```python
from build123d import *

# Parameters (mm, degrees)
SKETCH1_W           = 15
SKETCH1_H           = 185.68
SKETCH1_R           = 2.895
SKETCH1_W_2         = 343.08
SKETCH1_H_2         = 25
SKETCH1_H_3         = 15
BOSS_EXTRUDE1_DEPTH = 8
SKETCH2_W           = 15
SKETCH2_H           = 10
BOSS_EXTRUDE2_DEPTH = 100
SKETCH3_R           = 2
BOSS_EXTRUDE3_DEPTH = 4
CUT_EXTRUDE1_REACH  = 367.547
SKETCH5_R           = 1.35
BOSS_EXTRUDE4_DEPTH = 5


with BuildPart() as part:
    # Sketch1 → Boss-Extrude1 (new body)
    # profile 1 of 11: a face of its own
    with BuildSketch(Plane(origin=(0, 0, 0), x_dir=(1, 0, 0), z_dir=(0, 1, 0))):
        with Locations((-7.5, 92.84)):
            Rectangle(SKETCH1_W, SKETCH1_H)
        with Locations(Location((-7.5, 6.7, 0), (0, 0, 270))):
            Circle(SKETCH1_R, mode=Mode.SUBTRACT)
        with Locations(Location((-7.5, 178.98, 0), (0, 0, 270))):
            Circle(SKETCH1_R, mode=Mode.SUBTRACT)
    # profile 2 of 11: a face of its own
    with BuildSketch(Plane(origin=(0, 0, 0), x_dir=(1, 0, 0), z_dir=(0, 1, 0))):
        with Locations((-32.89, 92.84)):
            Rectangle(SKETCH1_W, SKETCH1_H)
        with Locations(Location((-32.89, 6.7, 0), (0, 0, 270))):
            Circle(SKETCH1_R, mode=Mode.SUBTRACT)
        with Locations(Location((-32.89, 178.98, 0), (0, 0, 270))):
            Circle(SKETCH1_R, mode=Mode.SUBTRACT)
    # profile 3 of 11: a face of its own
    with BuildSketch(Plane(origin=(0, 0, 0), x_dir=(1, 0, 0), z_dir=(0, 1, 0))):
        with Locations((-72.88, 92.84)):
            Rectangle(SKETCH1_W, SKETCH1_H)
        with Locations(Location((-72.88, 6.7, 0), (0, 0, 270))):
            Circle(SKETCH1_R, mode=Mode.SUBTRACT)
        with Locations(Location((-72.88, 178.98, 0), (0, 0, 270))):
            Circle(SKETCH1_R, mode=Mode.SUBTRACT)
    # profile 4 of 11: a face of its own
    with BuildSketch(Plane(origin=(0, 0, 0), x_dir=(1, 0, 0), z_dir=(0, 1, 0))):
        with Locations((-112.87, 92.84)):
            Rectangle(SKETCH1_W, SKETCH1_H)
        with Locations(Location((-112.87, 6.7, 0), (0, 0, 270))):
            Circle(SKETCH1_R, mode=Mode.SUBTRACT)
        with Locations(Location((-112.87, 178.98, 0), (0, 0, 270))):
            Circle(SKETCH1_R, mode=Mode.SUBTRACT)
    # profile 5 of 11: a face of its own
    with BuildSketch(Plane(origin=(0, 0, 0), x_dir=(1, 0, 0), z_dir=(0, 1, 0))):
        with Locations((-157.74, 52.84)):
            Rectangle(SKETCH1_W_2, SKETCH1_H_2)
        with Locations(Location((-157.74, 52.84, 0), (0, 0, 270))):
            Circle(SKETCH1_R, mode=Mode.SUBTRACT)
    # profile 6 of 11: a face of its own
    with BuildSketch(Plane(origin=(0, 0, 0), x_dir=(1, 0, 0), z_dir=(0, 1, 0))):
        with Locations((-157.74, 92.84)):
            Rectangle(SKETCH1_W_2, SKETCH1_H_3)
        with Locations(Location((7.1, 92.84, 0), (0, 0, 270))):
            Circle(SKETCH1_R, mode=Mode.SUBTRACT)
        with Locations(Location((-157.74, 92.84, 0), (0, 0, 270))):
            Circle(SKETCH1_R, mode=Mode.SUBTRACT)
        with Locations(Location((-322.58, 92.84, 0), (0, 0, 270))):
            Circle(SKETCH1_R, mode=Mode.SUBTRACT)
    # profile 7 of 11: a face of its own
    with BuildSketch(Plane(origin=(0, 0, 0), x_dir=(1, 0, 0), z_dir=(0, 1, 0))):
        with Locations((-157.74, 132.84)):
            Rectangle(SKETCH1_W_2, SKETCH1_H_2)
        with Locations(Location((-157.74, 132.84, 0), (0, 0, 270))):
            Circle(SKETCH1_R, mode=Mode.SUBTRACT)
    # profile 8 of 11: a face of its own
    with BuildSketch(Plane(origin=(0, 0, 0), x_dir=(1, 0, 0), z_dir=(0, 1, 0))):
        with Locations((-202.61, 92.84)):
            Rectangle(SKETCH1_W, SKETCH1_H)
        with Locations(Location((-202.61, 178.98, 0), (0, 0, 270))):
            Circle(SKETCH1_R, mode=Mode.SUBTRACT)
        with Locations(Location((-202.61, 6.7, 0), (0, 0, 270))):
            Circle(SKETCH1_R, mode=Mode.SUBTRACT)
    # profile 9 of 11: a face of its own
    with BuildSketch(Plane(origin=(0, 0, 0), x_dir=(1, 0, 0), z_dir=(0, 1, 0))):
        with Locations((-242.6, 92.84)):
            Rectangle(SKETCH1_W, SKETCH1_H)
        with Locations(Location((-242.6, 178.98, 0), (0, 0, 270))):
            Circle(SKETCH1_R, mode=Mode.SUBTRACT)
        with Locations(Location((-242.6, 6.7, 0), (0, 0, 270))):
            Circle(SKETCH1_R, mode=Mode.SUBTRACT)
    # profile 10 of 11: a face of its own
    with BuildSketch(Plane(origin=(0, 0, 0), x_dir=(1, 0, 0), z_dir=(0, 1, 0))):
        with Locations((-282.59, 92.84)):
            Rectangle(SKETCH1_W, SKETCH1_H)
        with Locations(Location((-282.59, 178.98, 0), (0, 0, 270))):
            Circle(SKETCH1_R, mode=Mode.SUBTRACT)
        with Locations(Location((-282.59, 6.7, 0), (0, 0, 270))):
            Circle(SKETCH1_R, mode=Mode.SUBTRACT)
    # profile 11 of 11: a face of its own
    with BuildSketch(Plane(origin=(0, 0, 0), x_dir=(1, 0, 0), z_dir=(0, 1, 0))):
        with Locations((-307.98, 92.84)):
            Rectangle(SKETCH1_W, SKETCH1_H)
        with Locations(Location((-307.98, 178.98, 0), (0, 0, 270))):
            Circle(SKETCH1_R, mode=Mode.SUBTRACT)
        with Locations(Location((-307.98, 6.7, 0), (0, 0, 270))):
            Circle(SKETCH1_R, mode=Mode.SUBTRACT)
    extrude(amount=BOSS_EXTRUDE1_DEPTH)

    # Sketch2 → Boss-Extrude2 (add)
    with BuildSketch(Plane(origin=(0, 8, 0), x_dir=(1, 0, 0), z_dir=(0, 1, 0))):
        with Locations((6.3, 60.34)):
            Rectangle(SKETCH2_W, SKETCH2_H)
        with Locations((-73.7, 60.34)):
            Rectangle(SKETCH2_W, SKETCH2_H)
    extrude(amount=BOSS_EXTRUDE2_DEPTH)

    # Sketch3 → Boss-Extrude3 (add)
    with BuildSketch(Plane(origin=(0, 0, -65.34), x_dir=(-1, 0, 0), z_dir=(0, 0, -1))):
        with Locations(Location((-7.8, 103.1, 0), (0, 0, 180))):
            Circle(SKETCH3_R)
        with Locations(Location((-7.8, 26.15, 0), (0, 0, 180))):
            Circle(SKETCH3_R)
        with Locations(Location((72.2, 26.15, 0), (0, 0, 180))):
            Circle(SKETCH3_R)
        with Locations(Location((72.2, 103.1, 0), (0, 0, 180))):
            Circle(SKETCH3_R)
    extrude(amount=BOSS_EXTRUDE3_DEPTH)

    # Sketch5 → Cut-Extrude1 (cut, up to next)
    with BuildSketch(Plane(origin=(0, 0, -69.34), x_dir=(-1, 0, 0), z_dir=(0, 0, -1)), mode=Mode.PRIVATE) as cut_extrude1_sk1:
        with Locations((-7.8, 103.1)):
            Circle(SKETCH5_R)
    cut_extrude1_tool1 = extrude(cut_extrude1_sk1.sketch, amount=-CUT_EXTRUDE1_REACH, mode=Mode.PRIVATE) & part.part
    # Sketch5 → Cut-Extrude1 (cut, up to next)
    with BuildSketch(Plane(origin=(0, 0, -69.34), x_dir=(-1, 0, 0), z_dir=(0, 0, -1)), mode=Mode.PRIVATE) as cut_extrude1_sk2:
        with Locations((-7.8, 26.15)):
            Circle(SKETCH5_R)
    cut_extrude1_tool2 = extrude(cut_extrude1_sk2.sketch, amount=-CUT_EXTRUDE1_REACH, mode=Mode.PRIVATE) & part.part
    # Sketch5 → Cut-Extrude1 (cut, up to next)
    with BuildSketch(Plane(origin=(0, 0, -69.34), x_dir=(-1, 0, 0), z_dir=(0, 0, -1)), mode=Mode.PRIVATE) as cut_extrude1_sk3:
        with Locations((72.2, 26.15)):
            Circle(SKETCH5_R)
    cut_extrude1_tool3 = extrude(cut_extrude1_sk3.sketch, amount=-CUT_EXTRUDE1_REACH, mode=Mode.PRIVATE) & part.part
    # Sketch5 → Cut-Extrude1 (cut, up to next)
    with BuildSketch(Plane(origin=(0, 0, -69.34), x_dir=(-1, 0, 0), z_dir=(0, 0, -1)), mode=Mode.PRIVATE) as cut_extrude1_sk4:
        with Locations((72.2, 103.1)):
            Circle(SKETCH5_R)
    cut_extrude1_tool4 = extrude(cut_extrude1_sk4.sketch, amount=-CUT_EXTRUDE1_REACH, mode=Mode.PRIVATE) & part.part
    add(cut_extrude1_tool1.solids().sort_by_distance((7.8, 103.1, -69.34))[0], mode=Mode.SUBTRACT)
    add(cut_extrude1_tool2.solids().sort_by_distance((7.8, 26.15, -69.34))[0], mode=Mode.SUBTRACT)
    add(cut_extrude1_tool3.solids().sort_by_distance((-72.2, 26.15, -69.34))[0], mode=Mode.SUBTRACT)
    add(cut_extrude1_tool4.solids().sort_by_distance((-72.2, 103.1, -69.34))[0], mode=Mode.SUBTRACT)

    # Sketch7 → Boss-Extrude4 (add)
    with BuildSketch(Plane.ZY.offset(1.2)):
        Polygon((-40.34, 8), (-55.34, 108), (-55.34, 8), align=None)
    extrude(amount=-BOSS_EXTRUDE4_DEPTH)


solid = part.part
```
Geometry check sheet. Reference: the model listing, model coordinates, mm. A direction names the side the tool comes from. Round coordinates to 2 decimals unless told otherwise and drop trailing zeros. Loops run counter-clockwise (first coordinate to the right, second up) from the corner with the lowest first, then second, coordinate; pieces in that order, holes last. Notation, with made-up numbers: (56, 57.5) -> (70, 57.5) arc R27 cw to (70, 73.5) -> close; hole circle Ø1 at (19.25, 23.5). An arc over 180 degrees is marked (long way). Use a Markdown table: item, result.
(1) Sectioned sample at B-B (z = -158.5). Give the number of separate pieces and of enclosed holes in the cut face, then the cut area to 3 significant figures.
Calculated:
| item | result |
|---|---|
| separate pieces | 8 |
| enclosed holes | 0 |
| area | 960 mm² |
(2) Go/stop test with flat-tipped pins: P1, Ø4, axis at x = -151, y = 5.5, coming from the -Z side; P2, Ø4.5, axis at x = 8, y = 102.5, coming from the -Z side; P3, Ø4, axis at x = -144.5, y = 3.5, coming from the +Z side. Record where each tip stops, or that it passes through.
Calculated:
| item | result |
|---|---|
| P1 | z = -145.34 |
| P2 | z = -69.34 |
| P3 | z = -40.34 |
(3) Scan lines: probe 1 along Y at (x, z) = (-72, -62); probe 2 along Z at (x, y) = (-157.74, 6.25) (3 decimals); probe 3 along X at (y, z) = (4.75, -92.84) (3 decimals). Record each from-to range of solid material in increasing order.
Calculated:
| item | result |
|---|---|
| probe 1 | 0 to 24.81, 27.49 to 101.76, 104.44 to 108 |
| probe 2 | -145.34 to -135.735, -129.945 to -120.34, -100.34 to -95.735, -89.945 to -85.34, -65.34 to -55.735, -49.945 to -40.34 |
| probe 3 | -329.28 to -325.475, -319.685 to -160.635, -154.845 to 4.205, 9.995 to 13.8 |
(4) Sectioned sample at C-C (x = -93). Enter the section's corners in (y, z).
Calculated:
| item | result |
|---|---|
| outline | (0, -145.34) -> (8, -145.34) -> (8, -120.34) -> (0, -120.34) -> close; (0, -100.34) -> (8, -100.34) -> (8, -85.34) -> (0, -85.34) -> close; (0, -65.34) -> (8, -65.34) -> (8, -40.34) -> (0, -40.34) -> close |
(5) Set-up check for faces 1 (the flat face through (-105.37, 4, -110)), 2 (the flat face through (-93, 4, -40.34)), 3 (the flat face through (-66.2, 57, -60)): record each of +Z, -Z, +X, -X, +Y, -Y from which the full face is reachable in a straight line by a thin tool's end or side.
Calculated:
| item | result |
|---|---|
| face 1 | +Y, -Y |
| face 2 | +Z, +Y, -Y |
| face 3 | +Z, -Z, +Y |
(6) Mould release check, pull along Z, two halves, no side actions. Record for faces 4 (the flat face through (-80.38, 4, -75)), 5 (the flat face through (-113, 4, 0)), 6 (the flat face through (-73, 4, -185.68)), 7 (the flat face through (-93, 4, -85.34)): released by +Z, released by -Z, zero draft, split by the parting line, or undercut.
Calculated:
| item | result |
|---|---|
| face 4 | undercut |
| face 5 | released by +Z |
| face 6 | released by -Z |
| face 7 | undercut |
(7) Sectioned sample at A-A (y = 16). Enter the section's corners in (x, z), then the cut area to 3 significant figures.
Calculated:
| item | result |
|---|---|
| outline | (-81.2, -65.34) -> (-66.2, -65.34) -> (-66.2, -55.34) -> (-81.2, -55.34) -> close; (-1.2, -65.34) -> (13.8, -65.34) -> (13.8, -55.34) -> (3.8, -55.34) -> (3.8, -41.54) -> (-1.2, -41.54) -> close |
| area | 369 mm² |
(8) Sectioned sample at D-D (y = 61). Enter the section's corners in (x, z), then the cut area to 3 significant figures.
Calculated:
| item | result |
|---|---|
| outline | (-81.2, -65.34) -> (-66.2, -65.34) -> (-66.2, -55.34) -> (-81.2, -55.34) -> close; (-1.2, -65.34) -> (13.8, -65.34) -> (13.8, -55.34) -> (3.8, -55.34) -> (3.8, -48.29) -> (-1.2, -48.29) -> close |
| area | 335 mm² |
